```python
from build123d import *

# Parameters (mm, degrees)
BOSS_EXTRUDE1_DEPTH = 12.1700036
SKETCH2_W           = 8.1000092
SKETCH2_H           = 10.8000038
SKETCH2_W_2         = 6.0000134
SKETCH2_H_2         = 9.5240094
CUT_EXTRUDE1_DEPTH  = 3.999992
CUT_EXTRUDE2_DEPTH  = 10.1700076
CUT_EXTRUDE3_DEPTH  = 4.0060118
CUT_EXTRUDE4_DEPTH  = 4.6199806
CUT_EXTRUDE5_DEPTH  = 5.2500022
CUT_EXTRUDE6_REACH  = 83.189
SKETCH7_R           = 1.7499965
CUT_EXTRUDE7_DEPTH  = 2.2999954
CUT_EXTRUDE8_DEPTH  = 2.2999954
SKETCH10_R          = 1.2499975
CUT_EXTRUDE9_DEPTH  = 71.298530747


with BuildPart() as part:
    # Sketch1 → Boss-Extrude1 (new body)
    with BuildSketch(Plane(origin=(0, 0, 0), x_dir=(1, 0, 0), z_dir=(0, 1, 0))):
        Polygon((-26.1999984, 16.3249991), (-26.1999984, 23.4500039), (26.1999984, 23.4500039), (26.1999984, -23.4500039), (-26.1999984, -23.4500039), (-26.1999984, -16.3249991), (-65.1450056, -16.3249991), (-65.1450056, 16.3249991), align=None)
    extrude(amount=BOSS_EXTRUDE1_DEPTH)

    # Sketch2 → Cut-Extrude1 (cut)
    with BuildSketch(Plane(origin=(0, 12.1700036, 0), x_dir=(1, 0, 0), z_dir=(0, 1, 0))):
        with Locations((22.1499938, -18.050002)):
            Rectangle(SKETCH2_W, SKETCH2_H)
        with Locations((-62.1449989, -11.5629944)):
            Rectangle(SKETCH2_W_2, SKETCH2_H_2)
    extrude(amount=-CUT_EXTRUDE1_DEPTH, mode=Mode.SUBTRACT)

    # Sketch3 → Cut-Extrude2 (cut)
    with BuildSketch(Plane(origin=(0, 12.1700036, 0), x_dir=(1, 0, 0), z_dir=(0, 1, 0))):
        Polygon((-59.1449922, -12.2549793), (-35.6249986, -12.2549793), (-35.6249986, 5.9090179), (-30.9599838, 5.9090179), (-30.9599838, 8.9190195), (-35.6249986, 8.9190195), (-35.6249986, 11.7050185), (-59.1449922, 11.7050185), (-59.1449922, 8.9190195), (-63.810007, 8.9190195), (-63.810007, 5.9090179), (-59.1449922, 5.9090179), align=None)
        Polygon((18.0999892, -20.6560039), (-22.0000068, -20.6560039), (-22.0000068, 7.6439903), (-28.7650174, 7.6439903), (-28.7650174, 10.6439843), (-22.0000068, 10.6439843), (-22.0000068, 19.4439921), (18.0999892, 19.4439921), (18.0999892, 10.6439843), (24.8649998, 10.6439843), (24.8649998, 7.6439903), (18.0999892, 7.6439903), align=None)
    extrude(amount=-CUT_EXTRUDE2_DEPTH, mode=Mode.SUBTRACT)

    # Sketch4 → Cut-Extrude3 (cut)
    with BuildSketch(Plane(origin=(0, 0, -23.4500039), x_dir=(-1, 0, 0), z_dir=(0, 0, -1))):
        with BuildLine():
            Line((-1.1299952, 12.1700036), (-14.7299934, 12.1700036))
            ThreePointArc((-14.7299934, 12.1700036), (-7.9299943, 5.3700045), (-1.1299952, 12.1700036))
        make_face()
    extrude(amount=-CUT_EXTRUDE3_DEPTH, mode=Mode.SUBTRACT)

    # Sketch5 → Cut-Extrude4 (cut)
    with BuildSketch(Plane(origin=(0, 0, -16.3249991), x_dir=(-1, 0, 0), z_dir=(0, 0, -1))):
        with BuildLine():
            ThreePointArc((46.838108, 8.4362036), (54.615256842, 5.524304205), (59.595004, 12.1700036))
            Line((59.595004, 12.1700036), (46.838108, 12.1700036))
            Line((46.838108, 12.1700036), (42.7449996, 12.1700036))
            ThreePointArc((42.7449996, 12.1700036), (43.96774198, 9.400015303), (46.838108, 8.4362036))
        make_face()
    extrude(amount=-CUT_EXTRUDE4_DEPTH, mode=Mode.SUBTRACT)

    # Sketch6 → Cut-Extrude5 (cut)
    with BuildSketch(Plane(origin=(0, 12.1700036, 0), x_dir=(1, 0, 0), z_dir=(0, 1, 0))):
        Polygon((-62.6450106, 14.2591155), (-64.320008607, 13.29205495), (-64.320008607, 11.35793385), (-62.6450106, 10.3908733), (-60.970012593, 11.35793385), (-60.970012593, 13.29205495), align=None)
        Polygon((-62.6450106, -2.3908893), (-64.320008607, -3.35794985), (-64.320008607, -5.29207095), (-62.6450106, -6.2591315), (-60.970012593, -5.29207095), (-60.970012593, -3.35794985), align=None)
        Polygon((23.2000044, 21.3841203), (21.525006393, 20.41705975), (21.525006393, 18.48293865), (23.2000044, 17.5158781), (24.875002407, 18.48293865), (24.875002407, 20.41705975), align=None)
        Polygon((23.2000044, -6.7158743), (21.525006393, -7.68293485), (21.525006393, -9.61705595), (23.2000044, -10.5841165), (24.875002407, -9.61705595), (24.875002407, -7.68293485), align=None)
    extrude(amount=-CUT_EXTRUDE5_DEPTH, mode=Mode.SUBTRACT)

    # Cut-Extrude6: up to this face of the body (flat: up to its plane)
    cut_extrude6_end = Plane(part.part.faces().sort_by_distance((-47.3849954, 7.0849998, 12.2549793))[0])
    # Sketch7 → Cut-Extrude6 (cut, up to the picked face)
    with BuildSketch(Plane.XY.offset(23.4500039), mode=Mode.PRIVATE) as cut_extrude6_sk1:
        with Locations((-52.6700115, 12.1700036)):
            Circle(SKETCH7_R)
    cut_extrude6_tool1 = split(extrude(cut_extrude6_sk1.sketch, amount=-CUT_EXTRUDE6_REACH, mode=Mode.PRIVATE), bisect_by=cut_extrude6_end, keep=Keep.BOTH, mode=Mode.PRIVATE)
    # Sketch7 → Cut-Extrude6 (cut, up to the picked face)
    with BuildSketch(Plane.XY.offset(23.4500039), mode=Mode.PRIVATE) as cut_extrude6_sk2:
        with Locations((7.9299943, 12.1700036)):
            Circle(SKETCH7_R)
    cut_extrude6_tool2 = split(extrude(cut_extrude6_sk2.sketch, amount=-CUT_EXTRUDE6_REACH, mode=Mode.PRIVATE), bisect_by=cut_extrude6_end, keep=Keep.BOTH, mode=Mode.PRIVATE)
    add(cut_extrude6_tool1.solids().sort_by(Axis((-52.670012, 12.170004, 23.450004), (0, 0, -1)))[0], mode=Mode.SUBTRACT)
    add(cut_extrude6_tool2.solids().sort_by(Axis((7.929994, 12.170004, 23.450004), (0, 0, -1)))[0], mode=Mode.SUBTRACT)

    # Sketch8 → Cut-Extrude7 (cut)
    with BuildSketch(Plane(origin=(0, 0, 20.6560039), x_dir=(-1, 0, 0), z_dir=(0, 0, -1))):
        Polygon((-10.8799884, 12.1700036), (-10.8799884, 10.466832), (-7.9299943, 8.763634463), (-4.9800002, 10.466832), (-4.9800002, 12.1700036), align=None)
    extrude(amount=-CUT_EXTRUDE7_DEPTH, mode=Mode.SUBTRACT)

    # Sketch9 → Cut-Extrude8 (cut)
    with BuildSketch(Plane(origin=(0, 0, 12.2549793), x_dir=(-1, 0, 0), z_dir=(0, 0, -1))):
        Polygon((49.7200174, 12.1700036), (49.7200174, 10.466832), (52.6700115, 8.763634463), (55.6200056, 10.466832), (55.6200056, 12.1700036), align=None)
    extrude(amount=-CUT_EXTRUDE8_DEPTH, mode=Mode.SUBTRACT)

    # Sketch10 → Cut-Extrude9 (cut, through all)
    with BuildSketch(Plane(origin=(0, 12.1700036, 0), x_dir=(1, 0, 0), z_dir=(0, 1, 0))):
        with Locations(Location((-62.6450106, 12.3249944, 0), (0, 0, 270))):
            Circle(SKETCH10_R)
        with Locations(Location((-62.6450106, -4.3250104, 0), (0, 0, 270))):
            Circle(SKETCH10_R)
        with Locations(Location((23.2000044, -8.6499954, 0), (0, 0, 270))):
            Circle(SKETCH10_R)
        with Locations(Location((23.2000044, 19.4499992, 0), (0, 0, 270))):
            Circle(SKETCH10_R)
    extrude(amount=-CUT_EXTRUDE9_DEPTH, mode=Mode.SUBTRACT)


solid = part.part
```
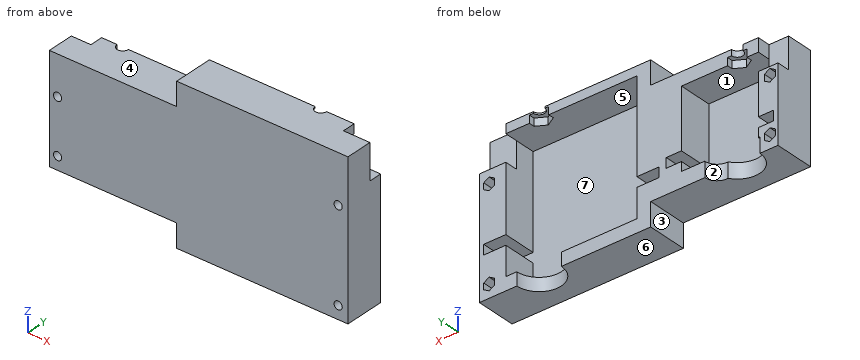
Read the model definition and answer for the solid it produces. Units are mm, in the model's axes. Face numbers are marked on the shaded views. A direction names the side the tool comes from. Coordinates: 2 decimals unless noted, no trailing zeros. Loops run counter-clockwise (first coordinate to the right, second up) from the corner with the lowest first, then second, coordinate; pieces in that order, holes last.
(1) The part is cut by section B-B (x = -5). Determine the outline of the cut face in (y, z), and give its area (3 significant figures).
Solution:
outline: (0, -23.45) - (12.17, -23.45) - (12.17, -19.44) - (2, -19.44) - (2, 20.66) - (12.17, 20.66) - (12.17, 23.45) - (0, 23.45) - close
area: 163 mm2
(2) A tool of negligible diameter and unlimited length cuts with its end or side. For the marked faces 1, 2 and 3, from which of +Z, -Z, +X, -X, +Y, -Y can it reach the whole face along a straight path? Write none if from no direction.
Solution:
face 1: +Y
face 2: -Z, +Y
face 3: -Z, -X, +Y, -Y
(3) The part is cut by section A-A (z = -2). Determine the outline of the cut face in (x, y) (3 decimals).
Solution:
outline: (-65.145, 0) - (26.2, 0) - (26.2, 12.17) - (18.1, 12.17) - (18.1, 2) - (-22, 2) - (-22, 12.17) - (-35.625, 12.17) - (-35.625, 2) - (-59.145, 2) - (-59.145, 12.17) - (-65.145, 12.17) - close
(4) Flat-ended cylindrical pins translate along their axes: pin 1 Ø2.5 at (x, y) = (-32.5, 6.5) entering from +Z (3 decimals); pin 2 Ø4.5 at (y, z) = (11, 14) entering from -X (3 decimals); pin 3 Ø6 at (x, y) = (-50.5, 4) entering from -Z (3 decimals); pin 4 Ø2.5 at (x, z) = (23.5, 8) entering from +Y. Find the tip coordinate at first contact, or state that the pin passes through.
Solution:
pin 1: stops at z = 16.325
pin 2: stops at x = -59.145
pin 3: stops at z = -16.325
pin 4: stops at y = 12.17
(5) The mould has two halves that part along Z. Classify the marked faces 4, 5, 6 and 7: released by +Z, released by -Z, zero draft, split by the parting line, or undercut.
Solution:
face 4: released by +Z
face 5: undercut
face 6: released by -Z
face 7: undercut
(6) Consider line 1 along X through (y, z) = (10.25, -8) (3 decimals); line 2 along Z through (x, y) = (-40.5, 7.75) (3 decimals); line 3 along X through (y, z) = (10.75, 9) (3 decimals). Determine where each line is inside the solid, lowest interval first.
Solution:
line 1: x = -65.145 to -63.81, -30.96 to -28.765, 24.865 to 26.2
line 2: z = -16.325 to -11.705, 12.255 to 16.325
line 3: x = -35.625 to -22, 18.1 to 21.525, 24.875 to 26.2
